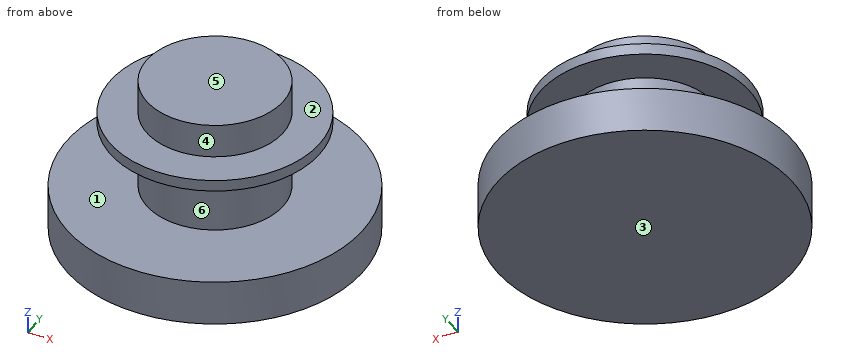
```python
from build123d import *

# Parameters (mm, degrees)
F0_R     = 6.5
F1_DEPTH = 2
F2_R     = 3
F3_DEPTH = 5
F5_R     = 4.593438
F6_DEPTH = 0.5


with BuildPart() as f1:
    # F0 (on Top) → F1 (new body)
    with BuildSketch(Plane.XY):
        Circle(F0_R)
    extrude(amount=F1_DEPTH)

    # F2 (on face) → F3 (join)
    with BuildSketch(Plane.XY.offset(2)):
        Circle(F2_R)
    extrude(amount=F3_DEPTH)

    # F5 (on offset) → F6 (join)
    with BuildSketch(Plane.XY.offset(5)):
        Circle(F5_R)
    extrude(amount=F6_DEPTH)


solid = f1.part
```
Here's how the part is built. I have some questions about the finished solid (model axes, mm). Face numbers are marked on the shaded views. A direction names the side the tool comes from. Give positions to 0.01 mm unless a question says otherwise; leave off trailing zeros. Write each loop counter-clockwise with the first axis right and the second up, starting at its lowest first coordinate (ties: lowest second). Pieces come first, ordered by that corner, then holes.
(1) On a 3-axis mill with a long thin cutter (end or side, diameter ignored), from which of +Z, -Z, +X, -X, +Y, -Y can I reach the whole of each face in a straight line? I mean the marked faces 4, 5 and 6. Say none if no direction works.
Output values:
face 4: +Z
face 5: +Z, +X, -X, +Y, -Y
face 6: none
(2) If I drill on L1, parallel to Z at x = 1, y = 3; L2, parallel to Z at x = -2.25, y = -4.25; L3, parallel to X at y = -0.75, z = 2.5, over which ranges is the centre line in solid material (lowest first)?
Output values:
L1: z = 0 to 2, 5 to 5.5
L2: z = 0 to 2
L3: x = -2.9 to 2.9
(3) Imagine slicing it at A-A, the plane y = 4.25. Write out the boundary of the cut face in (x, z), and give its area (3 significant figures).
Output values:
outline: (-4.92, 0) - (4.92, 0) - (4.92, 2) - (-4.92, 2) - close; (-1.74, 5) - (1.74, 5) - (1.74, 5.5) - (-1.74, 5.5) - close
area: 21.4 mm2
(4) Imagine slicing it at D-D, the plane z = 3.75. Write out the boundary of the cut face in (x, y).
Output values:
outline: circle Ø6 at (0, 0)
(5) Thinking about a two-plate mould opening in Z: for the marked faces 1, 2 and 3, which applies, pulls with the +Z half, pulls with the -Z half, needs draft (parallel to the pull), parting line crosses it, or undercut?
Output values:
face 1: undercut
face 2: pulls with the +Z half
face 3: pulls with the -Z half
(6) Imagine slicing it at B-B, the plane y = 0. Write out the boundary of the cut face in (x, z).
Output values:
outline: (-6.5, 0) - (6.5, 0) - (6.5, 2) - (3, 2) - (3, 5) - (4.59, 5) - (4.59, 5.5) - (3, 5.5) - (3, 7) - (-3, 7) - (-3, 5.5) - (-4.59, 5.5) - (-4.59, 5) - (-3, 5) - (-3, 2) - (-6.5, 2) - close
(7) Imagine slicing it at C-C, the plane x = -4. Write out the boundary of the cut face in (y, z).
Output values:
outline: (-5.12, 0) - (5.12, 0) - (5.12, 2) - (-5.12, 2) - close; (-2.26, 5) - (2.26, 5) - (2.26, 5.5) - (-2.26, 5.5) - close
(8) Will these pins go through, and if not, where does the flat tip stop? pin 1 (1.5 mm diameter, centred on y = 1, z = 3, fed in from +X); pin 2 (1 mm diameter, centred on x = 2.5, z = 3.5, fed in from -Y); pin 3 (2 mm diameter, centred on x = 2, y = 2.5, fed in from +Z); pin 4 (3 mm diameter, centred on x = -4.5, y = 3.5, fed in from +Z).
Output values:
pin 1: stops at x = 2.99
pin 2: stops at y = -2.24
pin 3: stops at z = 7
pin 4: stops at z = 5.5
